Autodesk Inventor part; units mm, degrees
ref_plane "YZ Plane" through (0, 0, 0) normal (1, 0, 0) x (0, 1, 0)
ref_plane "XZ Plane" through (0, 0, 0) normal (0, 1, 0) x (-1, 0, 0)
ref_plane "XY Plane" through (0, 0, 0) normal (0, 0, 1) x (1, 0, 0)
sketch "Sketch1" plane through (0, 0, 0) normal (0, 1, 0) x (-1, 0, 0)
  line L0 (0, 0) -> (220, 0)
  line L1 (220, 0) -> (220, -100)
  line L2 (220, -100) -> (0, -100)
  line L3 (0, -100) -> (0, 0)
  dimension "d0" = 220
  dimension "d1" = 100
extrude "Extrusion1" add sketch "Sketch1" along normal blind 200
sketch "Sketch2" plane through (0, 200, 0) normal (0, 1, 0) x (1, 0, 0)
  line L0 (-210, 5) -> (-10, 5)
  line L1 (-5, 10) -> (-5, 90)
  line L2 (-10, 95) -> (-210, 95)
  line L3 (-215, 90) -> (-215, 10)
  line L4 (-220, 100) -> (-220, 0)
  line L5 (0, 0) -> (0, 100)
  arc A0 (-210, 95) -> (-215, 90) centre (-210, 90) ccw
  arc A1 (-5, 90) -> (-10, 95) centre (-10, 90) ccw
  arc A2 (-10, 5) -> (-5, 10) centre (-10, 10) ccw
  arc A3 (-215, 10) -> (-210, 5) centre (-210, 10) ccw
  point P0 (-215, 5)
  point P1 (-5, 95)
  point P2 (-5, 5)
  point P3 (-215, 95)
  dimension "d4" = 5
  dimension "d5" = 5
  dimension "d6" = 5
  dimension "d7" = 5
  dimension "d8" = 5
extrude "Extrusion2" cut sketch "Sketch2" against normal blind 195
properties part number "balde"
Verification items for the finished model (mm, model axes). A direction names the side the tool comes from. Give positions to 0.01 mm unless a question says otherwise; leave off trailing zeros. Order: outer loops, then holes, each group sorted by start corner. A loop starts at its lowest first (then second) coordinate and runs counter-clockwise, first axis right, second up. Notation, with made-up numbers: M 66,76 L 124,76 A18 cw 124,98 Z; hole C 8,68 d9. An arc over 180 degrees is marked long. Return JSON: item names as keys, results as strings. Group by question number.
1) Section check A-A on y = 56.5. Record the cut outline in (x, z), and give its area (3 significant figures).
2) Section check B-B on z = -42. Record the cut outline in (x, y).
3) Section check C-C on x = -19.5. Record the cut outline in (y, z), and give its area (3 significant figures).
4) Access from +Z, -Z, +X, -X, +Y, -Y to the whole of each face (thin tool, end or side, straight path). Record for faces 1 (the face through (-6, 104, -93)), 2 (the face through (-108, 0, -49)).
5) Go/stop test with flat-tipped pins: pin 1 Ø6 at (x, z) = (-105, -72.5) entering from -Y; pin 2 Ø5 at (x, z) = (-61.5, -76) entering from +Y. Record where each tip stops, or that it passes through.
6) Scan lines: line 1 (X direction, y = 18.5, z = -83); line 2 (Z direction, x = -156, y = 145); line 3 (Y direction, x = -34, z = -87). Record each from-to range of solid material in increasing order.
7) Mould release check, pull along X, two halves, no side actions. Record for faces 3 (the face through (-112, 99, -100)), 4 (the face through (0, 99, -51)), 5 (the face through (-220, 99, -49)), 6 (the face through (-213, 104, -94)): pulls with the +X half, pulls with the -X half, needs draft (parallel to the pull), parting line crosses it, or undercut.
Answer block:
{
 "1": {"outline": "M -220,-100 L 0,-100 L 0,0 L -220,0 Z; hole M -215,-90 A5 ccw -210,-95 L -10,-95 A5 ccw -5,-90 L -5,-10 A5 ccw -10,-5 L -210,-5 A5 ccw -215,-10 Z", "area": "3,120 mm^2"},
 "2": {"outline": "M -220,0 L 0,0 L 0,200 L -5,200 L -5,5 L -215,5 L -215,200 L -220,200 Z"},
 "3": {"outline": "M 0,-100 L 200,-100 L 200,-95 L 5,-95 L 5,-5 L 200,-5 L 200,0 L 0,0 Z", "area": "2,450 mm^2"},
 "4": {"face 1": "+Y", "face 2": "+Z, -Z, +X, -X, -Y"},
 "5": {"pin 1": "stops at y = 0", "pin 2": "stops at y = 5"},
 "6": {"line 1": "x = -220 to -215, -5 to 0", "line 2": "z = -100 to -95, -5 to 0", "line 3": "y = 0 to 5"},
 "7": {"face 3": "needs draft", "face 4": "pulls with the +X half", "face 5": "pulls with the -X half", "face 6": "undercut"}
}
